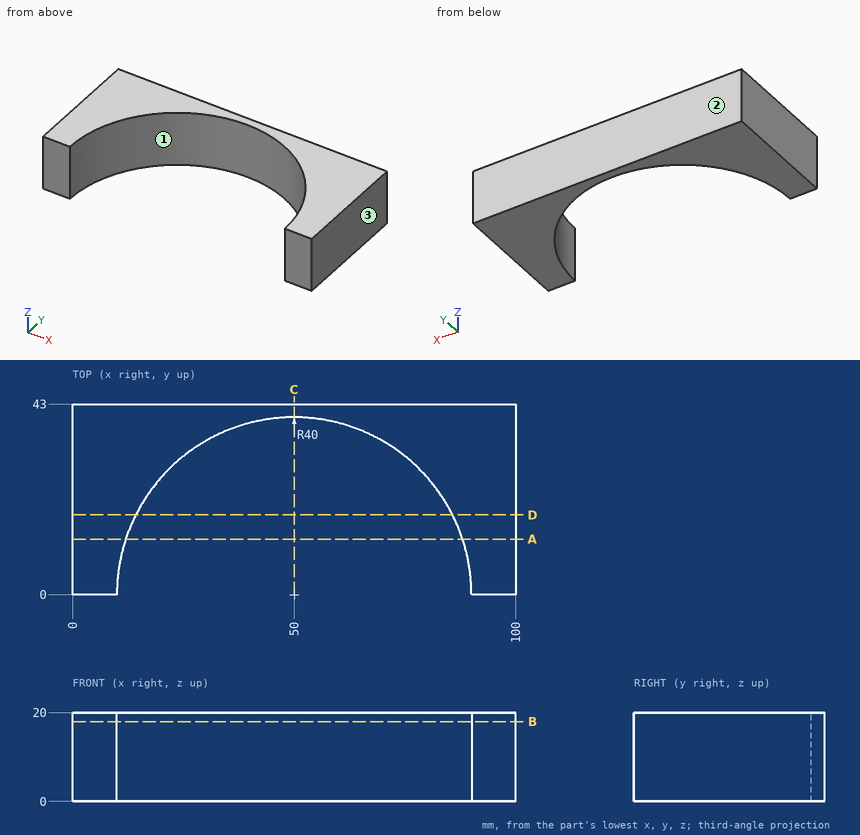
Can you work these out from the drawing? Everything is in mm from the part's minimum corner. Give positions to 0.01 mm unless a question says otherwise; leave off trailing zeros. Loops run counter-clockwise (first coordinate to the right, second up) from the corner with the lowest first, then second, coordinate; pieces in that order, holes last. Notation, with made-up numbers: (-8.75, -28) - (-3.75, -28) arc R27 ccw to (-3.75, -9) - close; hole circle Ø7 at (-15.75, -7.75). An arc over 180 degrees is marked (long way). Answer as a JSON object with one key per item and string values.
Q1. If I drill on L1, parallel to X at y = 12.5, z = 12.75; L2, parallel to X at y = 25.5, z = 10.25; L3, parallel to Y at x = 20.5, z = 19.25, over which ranges is the centre line in solid material (lowest first)?
Geometry says:
{"L1": "0 to 12, 88 to 100", "L2": "0 to 19.18, 80.82 to 100", "L3": "27.01 to 43"}
Q2. Imagine slicing it at A-A on y = 12.5. Write out the boundary of the cut face in (x, z).
Geometry says:
{"outline": "(0, 0) - (12, 0) - (12, 20) - (0, 20) - close; (88, 0) - (100, 0) - (100, 20) - (88, 20) - close"}
Q3. Imagine slicing it at B-B on z = 18. Write out the boundary of the cut face in (x, y), plus the area to 3 significant figures.
Geometry says:
{"outline": "(0, 0) - (10, 0) arc R40 cw to (90, 0) - (100, 0) - (100, 43) - (0, 43) - close", "area": "1,790 mm²"}
Q4. Imagine slicing it at C-C on x = 50. Write out the boundary of the cut face in (y, z), plus the area to 3 significant figures.
Geometry says:
{"outline": "(40, 0) - (43, 0) - (43, 20) - (40, 20) - close", "area": "60.0 mm²"}
Q5. Will these pins go through, and if not, where does the flat tip stop? P1, Ø1, axis at x = 84.5, z = 12.5, coming from the -Y side; P2, Ø3, axis at x = 59.5, z = 9.5, coming from the -Y side; P3, Ø1.5, axis at x = 23.5, z = 15, coming from the -Y side.
Geometry says:
{"P1": "y = 19.36", "P2": "y = 38.46", "P3": "y = 29.28"}
Q6. If we mould it in two halves opening along X, with no side actions, what happens to the marked faces 1, 2 and 3? For each: pulls with the +X half, pulls with the -X half, needs draft (parallel to the pull), parting line crosses it, or undercut.
Geometry says:
{"face 1": "undercut", "face 2": "needs draft", "face 3": "pulls with the +X half"}
Q7. Imagine slicing it at D-D on y = 18. Write out the boundary of the cut face in (x, z).
Geometry says:
{"outline": "(0, 0) - (14.28, 0) - (14.28, 20) - (0, 20) - close; (85.72, 0) - (100, 0) - (100, 20) - (85.72, 20) - close"}
